The model under review builds one solid part; all positions refer to its coordinate system, in mm. Round coordinates to 2 decimals unless told otherwise and drop trailing zeros. Loops run counter-clockwise (first coordinate to the right, second up) from the corner with the lowest first, then second, coordinate; pieces in that order, holes last. Notation, with made-up numbers: (-4.5, 62) -> (4.5, 62) arc R29 cw to (4.5, 87) -> close; hole circle Ø1 at (-18, 81.25). An arc over 180 degrees is marked (long way). Write each question's results on one line, items separated by ' | '. Start each with the question number.
Item 1: For L1, parallel to Z at x = -23, y = 28; L2, parallel to Y at x = 15.5, z = 59; L3, parallel to X at y = -5, z = 139, list the stretches that pass through material, from the lowest coordinate up. Write a range as from..to.
Item 2: We need section A-A (z = 112). Give the boundary of the cut face in (x, y), and give its area (3 significant figures).
Item 3: We need section B-B (z = 80.5). Give the boundary of the cut face in (x, y), and give its area (3 significant figures).
Item 4: Clearance check with flat-ended pins moving along their axes: pin 1 Ø1 at (x, z) = (-2, 61) entering from +Y; pin 2 Ø1 at (y, z) = (-11.5, 103.5) entering from -X; pin 3 Ø5 at (y, z) = (5.5, 22) entering from +X. State where each tip first meets the part, or that it passes through.
from build123d import *

# Parameters (mm, degrees)
F2_R = 4


with BuildPart() as f1:
    # F0 (on Front) → F1 (revolve)
    with BuildSketch(Plane.XZ):
        with BuildLine():
            Line((0, 180), (0, 0))
            Line((0, 0), (40, 0))
            ThreePointArc((40, 0), (32.538114, 25.815038), (37.575505, 52.210504))
            ThreePointArc((37.575505, 52.210504), (28.101816, 70.006211), (26.999903, 90.136381))
            ThreePointArc((26.999903, 90.136381), (16.82912, 121.500761), (21.415917, 154.152415))
            ThreePointArc((21.415917, 154.152415), (20.945571, 158.627031), (18.790591, 162.576649))
            ThreePointArc((18.790591, 162.576649), (17.424024, 171.425157), (20, 180))
            Line((20, 180), (0, 180))
        make_face()
    revolve(axis=Axis((0, 0, 49.245128), (0, 0, -1)))

    # F2
    f2_edges = [f1.edges().sort_by_distance(p)[0] for p in [
        (-37.575505, 0, 52.210504),
        (-26.999903, 0, 90.136381),
    ]]
    fillet(f2_edges, radius=F2_R)


solid = f1.part
Here are the results:
1) L1: z = 0..8, 48.98..53.85 | L2: y = -28.86..28.86 | L3: x = -16.67..16.67
2) outline: circle Ø36.58 at (0, 0) | area: 1,050 mm2
3) outline: circle Ø52.86 at (0, 0) | area: 2,190 mm2
4) pin 1: stops at y = 31.86 | pin 2: stops at x = -17.62 | pin 3: stops at x = 32.86
